from build123d import *

# Parameters (mm, degrees)
BOSS_EXTRUDE1_DEPTH = 53
BOSS_EXTRUDE2_DEPTH = 8
FILLET2_R           = 1
FILLET3_R           = 1


with BuildPart() as part:
    # Sketch2 → Boss-Extrude1 (new body)
    with BuildSketch(Plane.XY):
        Polygon((0, 0), (0, -4.48), (-3.992377111, -2.175), (-3.992377111, -13.825), (0, -11.52), (0, -19), (0, -219), (0, -226.48), (-3.992377111, -224.175), (-3.992377111, -235.825), (0, -233.52), (0, -238), (2.9, -238), (2.9, -230.541230437), (2.9, -7.458769563), (2.9, 0), align=None)
    extrude(amount=BOSS_EXTRUDE1_DEPTH)

    # Sketch3 → Boss-Extrude2 (add)
    with BuildSketch(Plane(origin=(0, 0, 0), x_dir=(0, 0, -1), z_dir=(1, 0, 0))):
        Polygon((0, -119), (0, -58.5), (-2.8, -58.5), (-2.8, -179.5), (0, -179.5), align=None)
    extrude(amount=-BOSS_EXTRUDE2_DEPTH)

    # Fillet2
    fillet2_edges = [part.edges().sort_by_distance(p)[0] for p in [
        (2.9, 0, 26.5),
        (2.9, -238, 26.5),
        (0, -238, 26.5),
        (0, 0, 26.5),
    ]]
    fillet(fillet2_edges, radius=FILLET2_R)

    # Fillet3
    fillet3_edges = [part.edges().sort_by_distance(p)[0] for p in [
        (-8, -179.5, 1.4),
        (-4, -179.5, 0),
        (-8, -119, 2.8),
        (-4, -179.5, 2.8),
        (-8, -58.5, 1.4),
        (-4, -58.5, 2.8),
        (-8, -119, 0),
        (-4, -58.5, 0),
    ]]
    fillet(fillet3_edges, radius=FILLET3_R)


solid = part.part
Model file for the job. Use its own axes, mm. A direction names the side the tool comes from. Give positions to 0.01 mm unless a question says otherwise; leave off trailing zeros. Write each loop counter-clockwise with the first axis right and the second up, starting at its lowest first coordinate (ties: lowest second). Pieces come first, ordered by that corner, then holes. Notation, with made-up numbers: (-19, 32.5) -> (-2, 32.5) arc R25 cw to (-2, 59.5) -> close; hole circle Ø1 at (-12.75, 16). An arc over 180 degrees is marked (long way). Write item = value, one per line.
(1) Slice it at D-D, the plane y = -47.5. Give the cut face in (x, z).
Determined:
outline = (0, 0) -> (2.9, 0) -> (2.9, 53) -> (0, 53) -> close
(2) Slice it at C-C, the plane x = -2.25. Give the cut face in (y, z), then the cut area to 3 significant figures.
Determined:
outline = (-234.82, 0) -> (-225.18, 0) -> (-225.18, 53) -> (-234.82, 53) -> close; (-179.5, 1) arc R1 ccw to (-178.5, 0) -> (-59.5, 0) arc R1 ccw to (-58.5, 1) -> (-58.5, 1.8) arc R1 ccw to (-59.5, 2.8) -> (-178.5, 2.8) arc R1 ccw to (-179.5, 1.8) -> close; (-12.82, 0) -> (-3.18, 0) -> (-3.18, 53) -> (-12.82, 53) -> close
area = 1,360 mm2
(3) Slice it at A-A, the plane y = -73. Give the cut face in (x, z), then the cut area to 3 significant figures.
Determined:
outline = (-8, 1) arc R1 ccw to (-7, 0) -> (2.9, 0) -> (2.9, 53) -> (0, 53) -> (0, 2.8) -> (-7, 2.8) arc R1 ccw to (-8, 1.8) -> close
area = 176 mm2
(4) Flat gauge pins, fed straight in: P1, Ø4, axis at x = -5, y = -160.5, coming from the +Z side; P2, Ø1, axis at y = -235, z = 36.5, coming from the -X side; P3, Ø1.5, axis at y = -169, z = 26, coming from the -X side. Where does each tip first touch, or does it go through?
Determined:
P1 = 2.8
P2 = -3.99
P3 = 0
(5) Mould opens along Y. For faces 1 (the face through (0, -117, 26)), 2 (the face through (-3.992, -230, 26)) say: released by +Y, released by -Y, zero draft, split by the parting line, or undercut.
Determined:
face_1 = undercut
face_2 = zero draft
(6) Probe line 1 along X through (y, z) = (-31, 27.5); line 2 along Y through (x, z) = (-2.75, 23.5); line 3 along Z through (x, y) = (-6, -132.5). List the from-to ranges inside material, lowest first.
Determined:
line_1 = 0 to 2.9
line_2 = -235.11 to -224.89, -13.11 to -2.89
line_3 = 0 to 2.8
(7) Tool access for faces 3 (the face through (2.9, -121, 26)), 4 (the face through (-3, -118, 2.8)): list every direction of +Z, -Z, +X, -X, +Y, -Y with a clear straight run to the whole face (end or side of a thin tool).
Determined:
face_3 = +Z, -Z, +X, +Y, -Y
face_4 = +Z, -X
(8) Slice it at B-B, the plane z = 10.5. Give the cut face in (x, y) (3 decimals), then the cut area to 3 significant figures.
Determined:
outline = (-3.992, -235.825) -> (0, -233.52) -> (0, -237) arc R1 ccw to (1, -238) -> (1.9, -238) arc R1 ccw to (2.9, -237) -> (2.9, -1) arc R1 ccw to (1.9, 0) -> (1, 0) arc R1 ccw to (0, -1) -> (0, -4.48) -> (-3.992, -2.175) -> (-3.992, -13.825) -> (0, -11.52) -> (0, -226.48) -> (-3.992, -224.175) -> close
area = 764 mm2
